Study the drawing (mm; zero at the part's minimum x, y, z) and answer. Give positions to 0.01 mm unless a question says otherwise; leave off trailing zeros. Order: outer loops, then holes, each group sorted by start corner. A loop starts at its lowest first (then second) coordinate and runs counter-clockwise, first axis right, second up. Notation, with made-up numbers: (-20, -3) -> (16, -3) arc R27 ccw to (16, 21) -> close; hole circle Ø1 at (-39, 88.25). An arc over 180 degrees is marked (long way). Use a Markdown table: item, result. Add a question column.
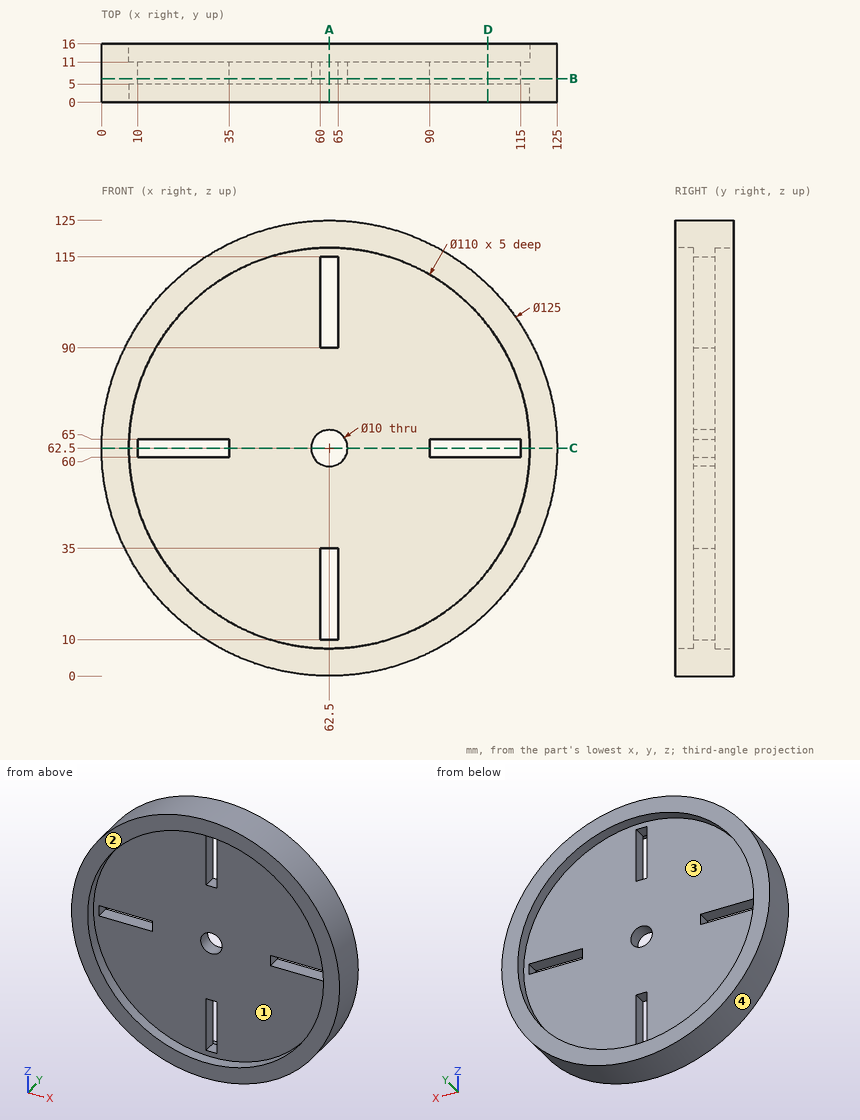
1) The part is cut by section D-D, the plane x = 106. Determine the outline of the cut face in (y, z), then the cut area to 3 significant figures.
2) Determine the mould class of the marked faces 1, 2, 3 and 4 for opening direction X: released by +X, released by -X, zero draft, split by the parting line, or undercut.
3) Flat-ended cylindrical pins translate along their axes: pin 1 (8 mm diameter, centred on x = 56.5, y = 13, fed in from -Z); pin 2 (5 mm diameter, centred on y = 4.5, z = 94.5, fed in from -X); pin 3 (1 mm diameter, centred on x = 83.5, y = 5.5, fed in from -Z). Find the tip coordinate at first contact, or state that the pin passes through.
4) The part is cut by section C-C, the plane z = 62.5. Determine the outline of the cut face in (x, y), then the cut area to 3 significant figures.
5) The part is cut by section B-B, the plane y = 6.5. Determine the outline of the cut face in (x, z).
6) Straight lines are drawn through the part: line 1 (Z direction, x = 62.5, y = 6.6); line 2 (X direction, y = 8.25, z = 62); line 3 (Z direction, x = 62.5, y = 14.9). For each, find the intervals that lie inside material, in ascending order.
7) The part is cut by section A-A, the plane x = 62.5. Determine the outline of the cut face in (y, z).
A:
| question | item | result |
|---|---|---|
| 1 | outline | (0, 17.62) -> (16, 17.62) -> (16, 28.84) -> (11, 28.84) -> (11, 60) -> (5, 60) -> (5, 28.84) -> (0, 28.84) -> close; (0, 96.16) -> (5, 96.16) -> (5, 65) -> (11, 65) -> (11, 96.16) -> (16, 96.16) -> (16, 107.38) -> (0, 107.38) -> close |
| 1 | area | 733 mm^2 |
| 2 | face 1 | undercut |
| 2 | face 2 | zero draft |
| 2 | face 3 | undercut |
| 2 | face 4 | split by the parting line |
| 3 | pin 1 | z = 0.03 |
| 3 | pin 2 | x = 7.4 |
| 3 | pin 3 | z = 3.46 |
| 4 | outline | (0, 0) -> (7.5, 0) -> (7.5, 5) -> (10, 5) -> (10, 11) -> (7.5, 11) -> (7.5, 16) -> (0, 16) -> close; (35, 5) -> (57.5, 5) -> (57.5, 11) -> (35, 11) -> close; (67.5, 5) -> (90, 5) -> (90, 11) -> (67.5, 11) -> close; (115, 5) -> (117.5, 5) -> (117.5, 0) -> (125, 0) -> (125, 16) -> (117.5, 16) -> (117.5, 11) -> (115, 11) -> close |
| 4 | area | 540 mm^2 |
| 5 | outline | circle Ø125 at (62.5, 62.5); hole (10, 60) -> (35, 60) -> (35, 65) -> (10, 65) -> close; hole circle Ø10 at (62.5, 62.5); hole (60, 10) -> (65, 10) -> (65, 35) -> (60, 35) -> close; hole (60, 90) -> (65, 90) -> (65, 115) -> (60, 115) -> close; hole (90, 60) -> (115, 60) -> (115, 65) -> (90, 65) -> close |
| 6 | line 1 | 0 to 10, 35 to 57.5, 67.5 to 90, 115 to 125 |
| 6 | line 2 | 0 to 10, 35 to 57.53, 67.47 to 90, 115 to 125 |
| 6 | line 3 | 0 to 7.5, 117.5 to 125 |
| 7 | outline | (0, 0) -> (16, 0) -> (16, 7.5) -> (11, 7.5) -> (11, 10) -> (5, 10) -> (5, 7.5) -> (0, 7.5) -> close; (0, 117.5) -> (5, 117.5) -> (5, 115) -> (11, 115) -> (11, 117.5) -> (16, 117.5) -> (16, 125) -> (0, 125) -> close; (5, 35) -> (11, 35) -> (11, 57.5) -> (5, 57.5) -> close; (5, 67.5) -> (11, 67.5) -> (11, 90) -> (5, 90) -> close |
